For this review, take the finished solid that the model builds, in its own axes (mm). Face numbers are marked on the shaded views. Coordinates: 2 decimals unless noted, no trailing zeros. Order: outer loops, then holes, each group sorted by start corner. A loop starts at its lowest first (then second) coordinate and runs counter-clockwise, first axis right, second up. Notation, with made-up numbers: (65, 82) -> (71, 82) arc R25 ccw to (71, 118) -> close; hole circle Ø3 at (30.25, 83.25). An arc over 180 degrees is marked (long way). Return JSON: item names as keys, results as strings. Group by question number.
Item 1: Insertion check: pin 1 (1.6 mm diameter, centred on x = -36, y = 2.5, fed in from -Z); pin 2 (1 mm diameter, centred on y = 2, z = -133.5, fed in from -X) (3 decimals); pin 3 (1 mm diameter, centred on x = 36.5, y = 2, fed in from +Z); pin 4 (5 mm diameter, centred on x = 30, z = 1.5, fed in from -Y). Each pin has a flat end and moves straight along its axis. Give the tip position at first contact, or say it passes through.
Item 2: For line 1 along Z through (x, y) = (-11.5, 0.25); line 2 along Z through (x, y) = (-21, 1.05) (3 decimals); line 3 along X through (y, z) = (2.8, -34.5) (3 decimals), list the stretches that pass through material, from the lowest coordinate up.
Item 3: Take a section at C-C (x = 27.5). Write out the cut boundary in (y, z) (3 decimals).
Item 4: Draft analysis for pull direction Y (two halves, no side actions). For the marked faces 1 and 2, state which applies: +Y half, -Y half, draft (parallel to the pull), parting line (faces both ways), or undercut.
Item 5: Take a section at A-A (x = -29.5). Write out the cut boundary in (y, z) (3 decimals).
Item 6: Take a section at B-B (z = 120.5). Write out the cut boundary in (x, y) (3 decimals).
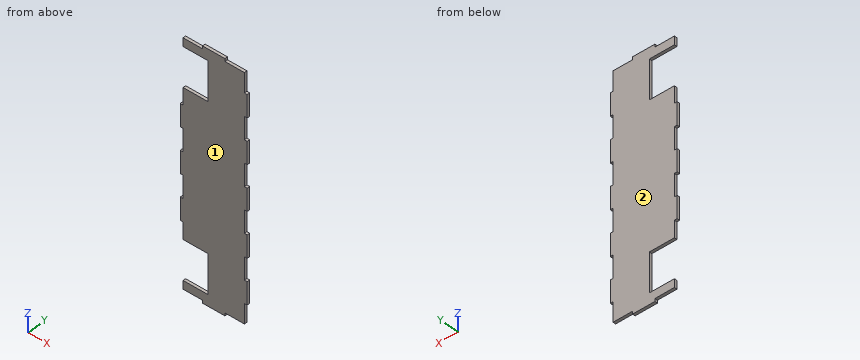
```python
from build123d import *

# Parameters (mm, degrees)
BOSS_EXTRUDE1_DEPTH     = 3.175
SKETCH2_W               = 31.75
SKETCH2_H               = 44.45
CUT_EXTRUDE1_DEPTH      = 1
CUT_EXTRUDE1_DEPTH_BACK = 4.175


with BuildPart() as part:
    # Sketch1 → Boss-Extrude1 (new body)
    with BuildSketch(Plane(origin=(0, 0, 0), x_dir=(1, 0, 0), z_dir=(0, 1, 0))):
        Polygon((0, 0), (-38.1, 0), (-38.1, 12.7), (-34.925, 12.7), (-34.925, 38.1), (-38.1, 38.1), (-38.1, 63.5), (-34.925, 63.5), (-34.925, 88.9), (-38.1, 88.9), (-38.1, 114.3), (-34.925, 114.3), (-34.925, 136.525), (-12.7, 136.525), (-12.7, 139.7), (0, 139.7), align=None)
    extrude(amount=BOSS_EXTRUDE1_DEPTH)

    # Mirror1: part across plane


with BuildPart() as part_1:
    add(part.part)
    add(part.part.mirror(Plane(origin=(0, 3.175, 0), x_dir=(0, 0, 1), z_dir=(-1, 0, 0))))

    # Sketch2 → Cut-Extrude1 (cut, two sides)
    with BuildSketch(Plane(origin=(0, 3.175, 0), x_dir=(1, 0, 0), z_dir=(0, 1, 0))) as cut_extrude1_sk:
        with Locations((-22.225, 104.775)):
            Rectangle(SKETCH2_W, SKETCH2_H)
    extrude(amount=CUT_EXTRUDE1_DEPTH, mode=Mode.SUBTRACT)
    extrude(cut_extrude1_sk.sketch, amount=-CUT_EXTRUDE1_DEPTH_BACK, mode=Mode.SUBTRACT)

    # Mirror2: part across plane


with BuildPart() as part_2:
    add(part_1.part)
    add(part_1.part.mirror(Plane(origin=(0, 3.175, 0), x_dir=(1, 0, 0), z_dir=(0, 0, 1))))


solid = part_2.part
```
Findings below:
{
 "1": {"pin 1": "stops at z = -63.5", "pin 2": "stops at x = -34.925", "pin 3": "stops at z = 114.3", "pin 4": "stops at y = 0"},
 "2": {"line 1": "z = -139.7 to -127, -82.55 to 82.55, 127 to 139.7", "line 2": "z = -136.525 to -127, -82.55 to 82.55, 127 to 136.525", "line 3": "x = -34.925 to 34.925"},
 "3": {"outline": "(0, -136.525) -> (3.175, -136.525) -> (3.175, 136.525) -> (0, 136.525) -> close"},
 "4": {"face 1": "-Y half", "face 2": "+Y half"},
 "5": {"outline": "(0, -136.525) -> (3.175, -136.525) -> (3.175, -127) -> (0, -127) -> close; (0, -82.55) -> (3.175, -82.55) -> (3.175, 82.55) -> (0, 82.55) -> close; (0, 127) -> (3.175, 127) -> (3.175, 136.525) -> (0, 136.525) -> close"},
 "6": {"outline": "(-6.35, 0) -> (34.925, 0) -> (34.925, 3.175) -> (-6.35, 3.175) -> close"}
}
